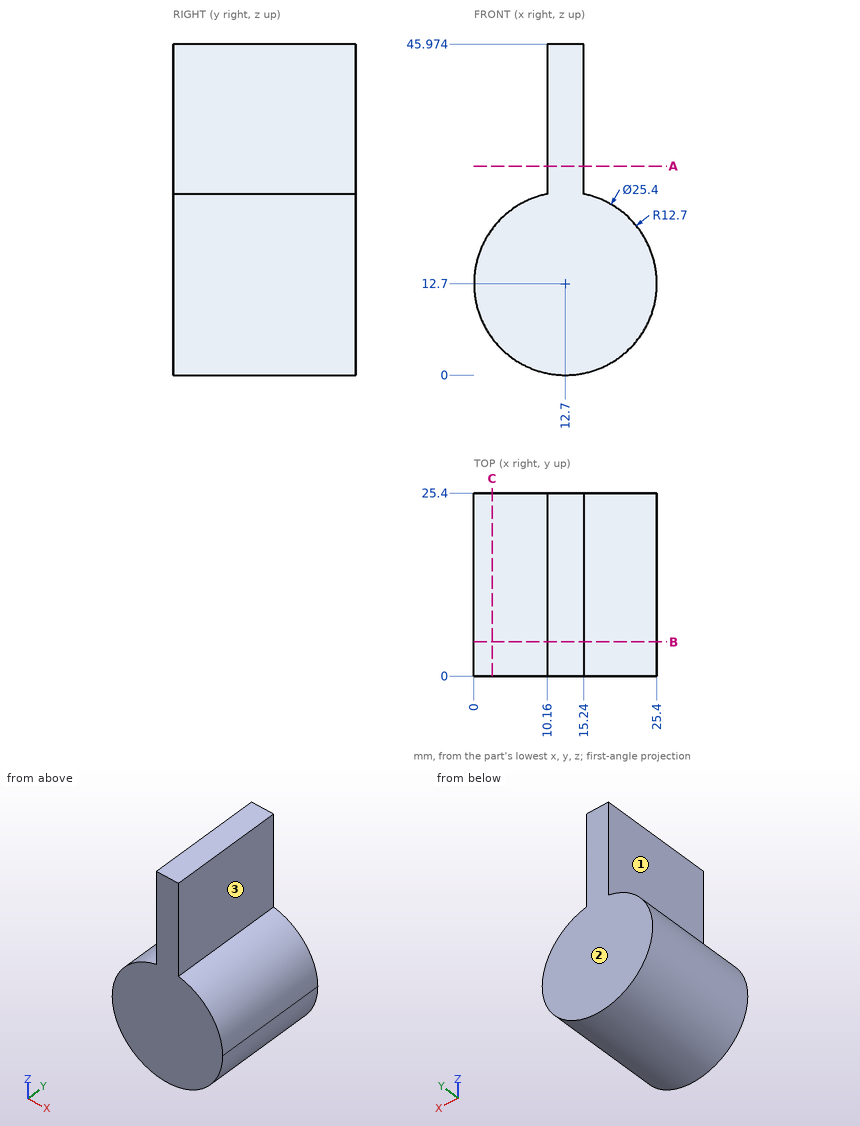
Study the drawing (mm; zero at the part's minimum x, y, z) and answer. A direction names the side the tool comes from. Round coordinates to 2 decimals unless told otherwise and drop trailing zeros. Write each loop counter-clockwise with the first axis right and the second up, starting at its lowest first coordinate (ties: lowest second). Pieces come first, ordered by that corner, then holes.
1) A cutting plane is placed at C-C (x = 2.5). Give the vertices of the cut face in (y, z), plus the area to 3 significant figures.
2) Given pin 1 Ø10 at (x, y) = (5.5, 12.5) entering from -Z; pin 2 Ø8 at (y, z) = (10.5, 24.5) entering from +X; pin 3 Ø8 at (x, z) = (7.5, 18) entering from -Y; pin 4 Ø6 at (y, z) = (8, 32.5) entering from -X, each flat-ended and moving along its own axis, determine where each tip first touches the part or whether it passes through.
3) A tool of negligible diameter and unlimited length cuts with its end or side. For the marked faces 1, 2 and 3, from which of +Z, -Z, +X, -X, +Y, -Y can it reach the whole face along a straight path? Write none if from no direction.
4) A cutting plane is placed at B-B (y = 4.75). Give the vertices of the cut face in (x, z).
5) Straight lines are drawn through the part: line 1 (Z direction, x = 12.25, y = 19); line 2 (X direction, y = 12.25, z = 41); line 3 (X direction, y = 11.25, z = 10). For each, find the intervals that lie inside material, in ascending order.
6) A cutting plane is placed at A-A (z = 29). Give the vertices of the cut face in (x, y).
Completed:
1. outline: (0, 5.13) - (25.4, 5.13) - (25.4, 20.27) - (0, 20.27) - close
1. area: 384 mm2
2. pin 1: stops at z = 0.19
2. pin 2: stops at x = 22.72
2. pin 3: stops at y = 0
2. pin 4: stops at x = 10.16
3. face 1: +Z, -X, +Y, -Y
3. face 2: +Z, -Z, +X, -X, +Y
3. face 3: +Z, +X, +Y, -Y
4. outline: (10.16, 25.14) arc R12.7 ccw (long way) to (15.24, 25.14) - (15.24, 45.97) - (10.16, 45.97) - close
5. line 1: z = 0.01 to 45.97
5. line 2: x = 10.16 to 15.24
5. line 3: x = 0.29 to 25.11
6. outline: (10.16, 0) - (15.24, 0) - (15.24, 25.4) - (10.16, 25.4) - close
